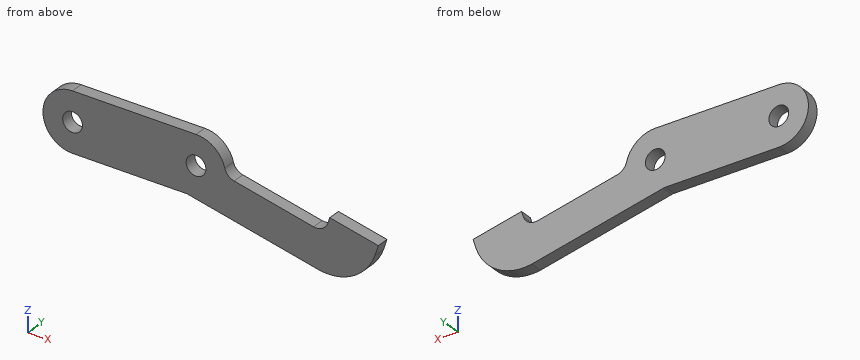
from build123d import *

# Parameters (mm, degrees)
SKETCH1_R           = 4
BOSS_EXTRUDE1_DEPTH = 5
FILLET1_R           = 5
SCALE1_SCALE        = 0.5


with BuildPart() as part:
    # Sketch1 → Boss-Extrude1 (new body)
    with BuildSketch(Plane(origin=(0, 0, 0), x_dir=(1, 0, 0), z_dir=(0, 1, 0))):
        with BuildLine():
            Line((0, 12), (46.309546143, 12))
            Line((46.309546143, 12), (100.107664183, 23.435142995))
            ThreePointArc((100.107664183, 23.435142995), (113.686830565, 20.974303457), (122.439553034, 10.304751439))
            Line((122.439553034, 10.304751439), (123.826560512, 6.023839123))
            Line((123.826560512, 6.023839123), (104.157567187, 1.843065531))
            Line((104.157567187, 1.843065531), (102, 8.502262467))
            Line((102, 8.502262467), (62, 0))
            ThreePointArc((62, 0), (58.485281374, -8.485281374), (50, -12))
            Line((50, -12), (0, -12))
            ThreePointArc((0, -12), (-12, 0), (0, 12))
        make_face()
        Circle(SKETCH1_R, mode=Mode.SUBTRACT)
        with Locations((50, 0)):
            Circle(SKETCH1_R, mode=Mode.SUBTRACT)
    extrude(amount=BOSS_EXTRUDE1_DEPTH)

    # Fillet1
    fillet1_edges = [part.edges().sort_by_distance(p)[0] for p in [
        (102, 2.5, -8.502262467),
        (62, 2.5, 0),
        (46.309546143, 2.5, -12),
    ]]
    fillet(fillet1_edges, radius=FILLET1_R)


with BuildPart() as part_1:
    # Scale1: scaled about (50.856755606, 2.5, -4.748712571)
    add(part.part.scale(SCALE1_SCALE).moved(Location((25.428377803, 1.25, -2.374356286))))


solid = part_1.part
Geometry: final body of the model. Coordinates: model frame, mm. Give positions to 0.01 mm unless a question says otherwise; leave off trailing zeros. Write each loop counter-clockwise with the first axis right and the second up, starting at its lowest first coordinate (ties: lowest second). Pieces come first, ordered by that corner, then holes.
(1) Cut plane A-A, the plane z = -1.75. Return loops of the section in (x, y), then the cut area to 3 significant figures.
(2) First-contact query: P1, Ø0.8, axis at x = 33, y = 2.5, coming from the -Z side. Flat tip, straight axial feed; report the tip coordinate or a pass-through.
(3) Cut plane C-C, the plane x = 40. Return loops of the section in (y, z), then the cut area to 3 significant figures.
(4) Cut plane B-B, the plane y = 2.35. Return loops of the section in (x, z) (1 decimal).
(5) Ray query, line 1 (X direction, y = 1.6, z = -1); line 2 (X direction, y = 3.65, z = -1.5); line 3 (Z direction, x = 51, y = 3.2). Return the intervals inside material, ascending.
(6) Cut plane D-D, the plane z = -13. Return loops of the section in (x, y), then the cut area to 3 significant figures.
Values follow:
1. outline: (19.46, 1.25) - (23.53, 1.25) - (23.53, 3.75) - (19.46, 3.75) - close; (27.33, 1.25) - (48.53, 1.25) - (48.53, 3.75) - (27.33, 3.75) - close; (52.33, 1.25) - (56.64, 1.25) - (56.64, 3.75) - (52.33, 3.75) - close
1. area: 73.9 mm2
2. P1: stops at z = -8.37
3. outline: (1.25, -8.37) - (3.75, -8.37) - (3.75, 3.63) - (1.25, 3.63) - close
3. area: 30.0 mm2
4. outline: (25.4, -8.4) - (48.3, -8.4) arc R2.5 cw to (48.8, -8.4) - (75.5, -14.1) arc R10 ccw to (86.6, -7.5) - (87.3, -5.4) - (77.5, -3.3) - (77.1, -4.5) arc R2.5 cw to (74.2, -6.2) - (58.2, -2.7) arc R2.5 cw to (56.2, -0.9) arc R6 ccw to (50.4, 3.6) - (25.4, 3.6) arc R6 ccw to start; hole circle Ø4 at (25.4, -2.4); hole circle Ø4 at (50.4, -2.4)
5. line 1: x = 19.59 to 23.98, 26.88 to 48.98, 51.88 to 56.27
5. line 2: x = 19.49 to 23.63, 27.23 to 48.63, 52.23 to 56.48
5. line 3: z = -8.89 to -4.29, -0.46 to 3.6
6. outline: (70.35, 1.25) - (82.03, 1.25) - (82.03, 3.75) - (70.35, 3.75) - close
6. area: 29.2 mm2
